Geometry check sheet. Reference: drawing and pictorial views, mm from the part's lowest x, y, z. Round coordinates to 2 decimals unless told otherwise and drop trailing zeros. Write each loop counter-clockwise with the first axis right and the second up, starting at its lowest first coordinate (ties: lowest second). Pieces come first, ordered by that corner, then holes. Notation, with made-up numbers: M -28,72.25 L 15,72.25 A18 ccw 15,81.25 Z; hole C 36.25,76 d3. An arc over 180 degrees is marked long. Answer in a Markdown table with one row per item. Add a question column.
1. Material ranges on probe 1 along Z at (x, y) = (237, 8.5); probe 2 along Z at (x, y) = (420.5, 11.75); probe 3 along X at (y, z) = (10.5, 12.5), recorded low to high.
2. Sectioned sample at B-B on x = 491. Record the cut outline in (y, z), plus the area to 3 significant figures.
3. Go/stop test with flat-tipped pins: pin 1 Ø2 at (y, z) = (10.5, 13.5) entering from -X; pin 2 Ø3 at (x, z) = (302, 11) entering from +Y; pin 3 Ø1 at (x, y) = (333, 14) entering from +Z; pin 4 Ø4 at (x, z) = (262.5, 6) entering from +Y. Record where each tip stops, or that it passes through.
4. Sectioned sample at A-A on y = 8. Record the cut outline in (x, z), plus the area to 3 significant figures.
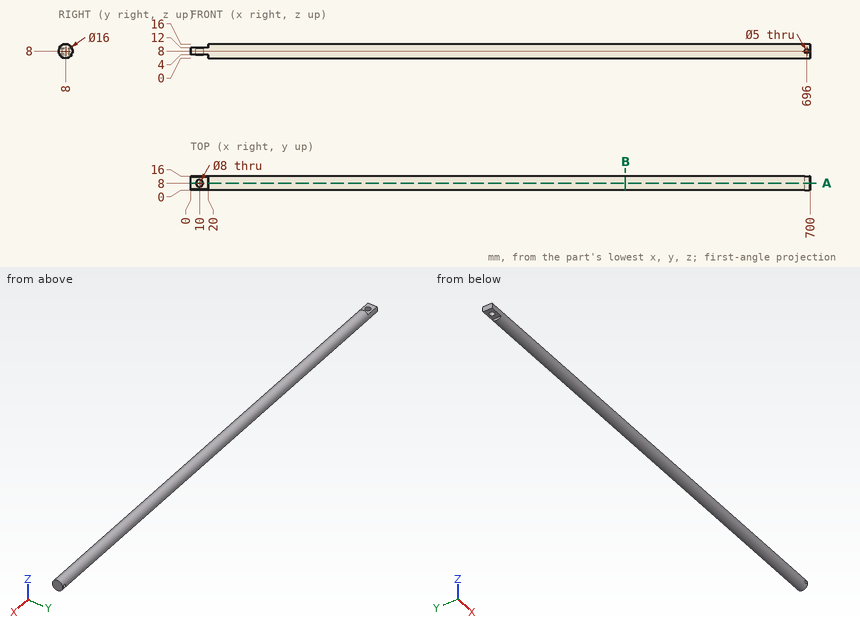
Geometry check:
| question | item | result |
|---|---|---|
| 1 | probe 1 | z = 0.02 to 15.98 |
| 1 | probe 2 | z = 0.93 to 15.07 |
| 1 | probe 3 | x = 20 to 700 |
| 2 | outline | C 8,8 d16 |
| 2 | area | 201 mm2 |
| 3 | pin 1 | stops at x = 20 |
| 3 | pin 2 | stops at y = 15.86 |
| 3 | pin 3 | stops at z = 13.81 |
| 3 | pin 4 | stops at y = 16 |
| 4 | outline | M 0,4 L 6,4 L 6,12 L 0,12 Z; M 14,4 L 20,4 L 20,0 L 700,0 L 700,16 L 20,16 L 20,12 L 14,12 Z; hole C 696,8 d5 |
| 4 | area | 11,000 mm2 |
